```python
from build123d import *

# Parameters (mm, degrees)
F0_R     = 6.5
F0_R_2   = 2.5
F1_DEPTH = 16
F2_DEPTH = 5.4


with BuildPart() as f1:
    # F0 (on Top) → F1 (new body)
    with BuildSketch(Plane.XY):
        Circle(F0_R)
        Polygon((-4.041452, 0), (-2.020726, 3.5), (2.020726, 3.5), (4.041452, 0), (2.020726, -3.5), (-2.020726, -3.5), align=None, mode=Mode.SUBTRACT)
        Polygon((2.020726, 3.5), (-2.020726, 3.5), (-4.041452, 0), (-2.020726, -3.5), (2.020726, -3.5), (4.041452, 0), align=None)
        Circle(F0_R_2, mode=Mode.SUBTRACT)
    extrude(amount=F1_DEPTH)

    # F0 (on Top) → F2 (cut)
    with BuildSketch(Plane.XY):
        Polygon((2.020726, 3.5), (-2.020726, 3.5), (-4.041452, 0), (-2.020726, -3.5), (2.020726, -3.5), (4.041452, 0), align=None)
        Circle(F0_R_2, mode=Mode.SUBTRACT)
    extrude(amount=F2_DEPTH, mode=Mode.SUBTRACT)


solid = f1.part
```
For this review, take the finished solid that the model builds, in its own axes (mm). A direction names the side the tool comes from. Give positions to 0.01 mm unless a question says otherwise; leave off trailing zeros. Write each loop counter-clockwise with the first axis right and the second up, starting at its lowest first coordinate (ties: lowest second). Pieces come first, ordered by that corner, then holes. Notation, with made-up numbers: M 24,55 L 31,55 A33 ccw 31,85 Z; hole C 40.25,43 d5. An arc over 180 degrees is marked long. One line per item, written item: value.
1) For line 1 (Y direction, x = 0, z = 11.5); line 2 (X direction, y = 2.5, z = 2); line 3 (X direction, y = -0.25, z = 12), list the stretches that pass through material, from the lowest coordinate up. Write a range as from..to.
Results are:
line 1: y = -6.5..-2.5, 2.5..6.5
line 2: x = -6..-2.6, 2.6..6
line 3: x = -6.5..-2.49, 2.49..6.5
2) Take a section at C-C, the plane y = 2.25. Write out the cut boundary in (x, z).
Results are:
outline: M -6.1,0 L -2.74,0 L -2.74,5.4 L -1.09,5.4 L -1.09,16 L -6.1,16 Z; M 1.09,5.4 L 2.74,5.4 L 2.74,0 L 6.1,0 L 6.1,16 L 1.09,16 Z
3) The part is to be moulded in two halves that separate along X. For faces 3 (the flat face through (3, -3, 0)), 4 (the cylindrical face through (-5.158, -3.955, 7.888)), 5 (the flat face through (3, 0, 5.4)), say which applies: +X half, -X half, draft (parallel to the pull), parting line (faces both ways), or undercut.
Results are:
face 3: draft
face 4: parting line
face 5: undercut
4) For P1, Ø2, axis at y = 5, z = 9.5, coming from the -X side; P2, Ø3, axis at x = 3, z = 6, coming from the -Y side; P3, Ø6, axis at x = 0, y = 0, coming from the -Z side, all flat-tipped, find the tip position at first contact; note any pin that passes through.
Results are:
P1: stops at x = -5.12
P2: stops at y = -6.32
P3: stops at z = 5.4
5) Take a section at A-A, the plane z = 4.25. Write out the cut boundary in (x, y).
Results are:
outline: C 0,0 d13; hole M -4.04,0 L -2.02,-3.5 L 2.02,-3.5 L 4.04,0 L 2.02,3.5 L -2.02,3.5 Z
6) Take a section at B-B, the plane x = 0. Write out the cut boundary in (y, z).
Results are:
outline: M -6.5,0 L -3.5,0 L -3.5,5.4 L -2.5,5.4 L -2.5,16 L -6.5,16 Z; M 2.5,5.4 L 3.5,5.4 L 3.5,0 L 6.5,0 L 6.5,16 L 2.5,16 Z
7) Take a section at D-D, the plane x = 2.75. Write out the cut boundary in (y, z), then the cut area to 3 significant figures.
Results are:
outline: M -5.89,0 L -2.24,0 L -2.24,5.4 L 2.24,5.4 L 2.24,0 L 5.89,0 L 5.89,16 L -5.89,16 Z
area: 164 mm²
8) For faces 1 (the flat face through (3, 0, 16)), 2 (the flat face through (0, -3.5, 3)), list the 3-axis set-ups (+Z, -Z, +X, -X, +Y, -Y) from which the entire face can be reached by the end or side of a thin tool; tool diameter is ignored.
Results are:
face 1: +Z, +X, -X, +Y, -Y
face 2: -Z
